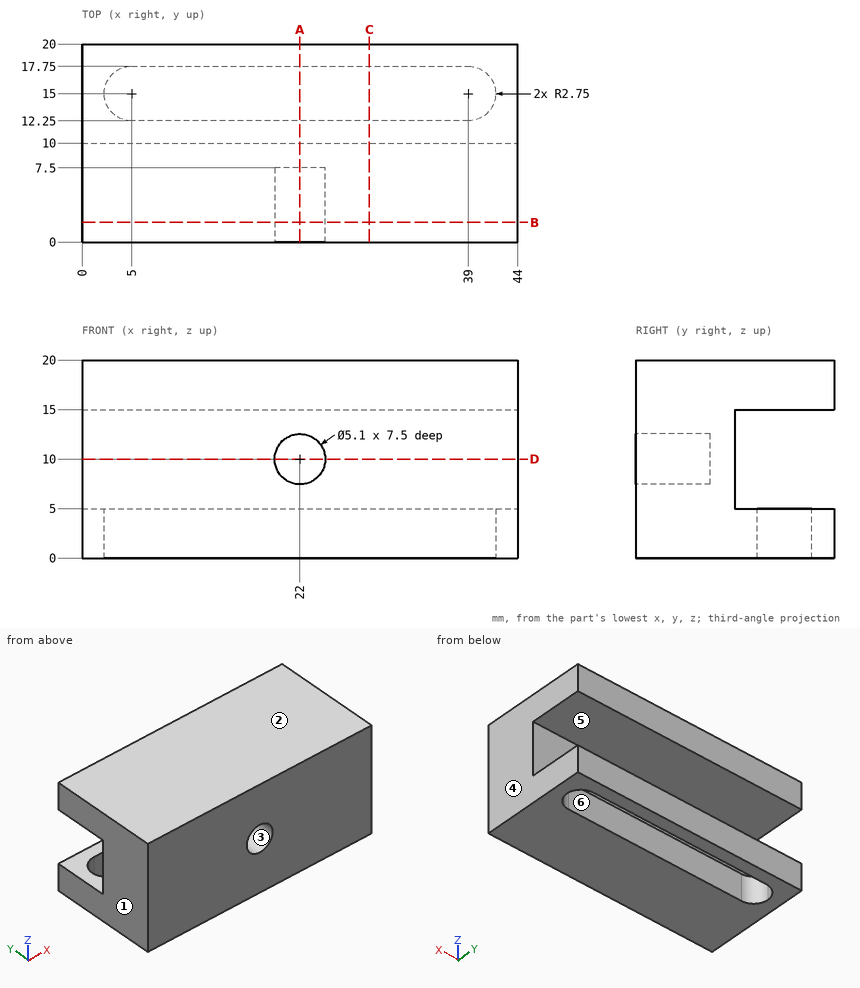
Job drawing, mm, ordinate dimensions from the low corner. One solid piece. A direction names the side the tool comes from. Give positions to 0.01 mm unless a question says otherwise; leave off trailing zeros. Loops run counter-clockwise (first coordinate to the right, second up) from the corner with the lowest first, then second, coordinate; pieces in that order, holes last. Notation, with made-up numbers: M 66,12.5 L 92,12.5 A14 cw 92,32.5 Z; hole C -22.75,75.25 d6. An arc over 180 degrees is marked long. Return JSON: item names as keys, results as strings.
1) Saw through at B-B, the plane y = 2. List the corners of the cut face in (x, z), then the cut area to 3 significant figures.
Calculated:
{"outline": "M 0,0 L 44,0 L 44,20 L 0,20 Z; hole C 22,10 d5.1", "area": "860 mm2"}
2) Saw through at C-C, the plane x = 29. List the corners of the cut face in (y, z), then the cut area to 4 significant figures.
Calculated:
{"outline": "M 0,0 L 12.25,0 L 12.25,5 L 10,5 L 10,15 L 20,15 L 20,20 L 0,20 Z; M 17.75,0 L 20,0 L 20,5 L 17.75,5 Z", "area": "272.5 mm2"}
3) Flat gauge pins, fed straight in: pin 1 Ø2.5 at (x, z) = (22, 11) entering from -Y; pin 2 Ø1 at (x, z) = (31, 8) entering from +Y; pin 3 Ø3 at (x, y) = (17.5, 15.5) entering from -Z. Where does each tip first touch, or does it go through?
Calculated:
{"pin 1": "stops at y = 7.5", "pin 2": "stops at y = 10", "pin 3": "stops at z = 15"}
4) Pull direction Z, two halves, no side cores. Call the marked faces 1, 2 and 3: released by +Z, released by -Z, zero draft, split by the parting line, or undercut.
Calculated:
{"face 1": "zero draft", "face 2": "released by +Z", "face 3": "undercut"}
5) Saw through at D-D, the plane z = 10. List the corners of the cut face in (x, y).
Calculated:
{"outline": "M 0,0 L 19.45,0 L 19.45,7.5 L 24.55,7.5 L 24.55,0 L 44,0 L 44,10 L 0,10 Z"}
6) Saw through at A-A, the plane x = 22. List the corners of the cut face in (y, z).
Calculated:
{"outline": "M 0,0 L 12.25,0 L 12.25,5 L 10,5 L 10,15 L 20,15 L 20,20 L 0,20 L 0,12.55 L 7.5,12.55 L 7.5,7.45 L 0,7.45 Z; M 17.75,0 L 20,0 L 20,5 L 17.75,5 Z"}
7) Drill centre lines: line 1 (X direction, y = 4.5, z = 10); line 2 (Z direction, x = 22, y = 4.75); line 3 (Z direction, x = 4.5, y = 11.25). Where is each one in solid material? Low to high.
Calculated:
{"line 1": "x = 0 to 19.45, 24.55 to 44", "line 2": "z = 0 to 7.45, 12.55 to 20", "line 3": "z = 0 to 5, 15 to 20"}
8) 3-axis set-ups, long thin cutter, end or side, ignore diameter. For the marked faces 4, 5 and 6: which of +Z, -Z, +X, -X, +Y, -Y reach the whole face in a straight line?
Calculated:
{"face 4": "+Z, -Z, +X, +Y, -Y", "face 5": "+X, -X, +Y", "face 6": "-Z"}
